Can you work these out from the model? Positions are in its coordinate system, mm. Face numbers are marked on the shaded views. A direction names the side the tool comes from. Coordinates: 2 decimals unless noted, no trailing zeros. Loops run counter-clockwise (first coordinate to the right, second up) from the corner with the lowest first, then second, coordinate; pieces in that order, holes last. Notation, with made-up numbers: (5.5, -0.5) -> (24.5, -0.5) arc R14 ccw to (24.5, 6.5) -> close; hole circle Ø1 at (29, -14). An arc over 180 degrees is marked (long way). Use one line per item in the form item = value. Start each with the question number.
(1) Imagine slicing it at B-B (y = 18). List the corners of the cut face in (x, z) for me, plus the area to 3 significant figures.
(2) Imagine slicing it at D-D (z = 17.5). List the corners of the cut face in (x, y) for me.
(3) Imagine slicing it at C-C (x = 33). List the corners of the cut face in (y, z) for me.
(4) On a 3-axis mill with a long thin cutter (end or side, diameter ignored), from which of +Z, -Z, +X, -X, +Y, -Y can I reach the whole of each face in a straight line? I mean the marked faces 1 and 2. Say none if no direction works.
(5) I need wall thicknesses on line 1 (X direction, y = 0.65, z = 33); line 2 (Z direction, x = 8, y = 1); line 3 (Y direction, x = 24.5, z = 29.5). Which ranges of each line are inside material? Lowest first, please. Write a range as [from, to].
(6) I'm going to push flat-ended pins straight in: pin 1 (10 mm diameter, centred on y = 14, z = 35.5, fed in from +X); pin 2 (5 mm diameter, centred on x = 33, z = 7, fed in from +Y); pin 3 (2.5 mm diameter, centred on x = 33, z = 33, fed in from -Y). Where does each tip first touch, or does it pass through?
(7) Imagine slicing it at A-A (z = 33). List the corners of the cut face in (x, y) for me.
```python
from build123d import *

# Parameters (mm, degrees)
EXTRUSION1_DEPTH = 40
ESQUISSE2_R      = 6.5
EXTRUSION2_DEPTH = 30
ESQUISSE3_R      = 1.5
EXTRUSION3_DEPTH = 30


with BuildPart() as part:
    # Esquisse1 → Extrusion1 (new body)
    with BuildSketch(Plane.XY):
        Polygon((0, 0), (0, 40), (1.5, 40), (1.5, 1.5), (40, 1.5), (40, 0), align=None)
    extrude(amount=EXTRUSION1_DEPTH)

    # Esquisse2 → Extrusion2 (cut)
    with BuildSketch(Plane(origin=(1.5, 0, 0), x_dir=(0, 0, -1), z_dir=(1, 0, 0))):
        with Locations(Location((-20, 18, 0), (0, 0, 90))):
            Circle(ESQUISSE2_R)
    extrude(amount=-EXTRUSION2_DEPTH, mode=Mode.SUBTRACT)

    # Esquisse3 → Extrusion3 (cut)
    with BuildSketch(Plane(origin=(0, 1.5, 0), x_dir=(-1, 0, 0), z_dir=(0, 1, 0))):
        with Locations(Location((-8.5, 33, 0), (0, 0, 90))):
            Circle(ESQUISSE3_R)
        with Locations(Location((-8.5, 7, 0), (0, 0, 90))):
            Circle(ESQUISSE3_R)
        with Locations(Location((-33, 7, 0), (0, 0, 90))):
            Circle(ESQUISSE3_R)
        with Locations(Location((-33, 33, 0), (0, 0, 90))):
            Circle(ESQUISSE3_R)
    extrude(amount=-EXTRUSION3_DEPTH, mode=Mode.SUBTRACT)


solid = part.part
```
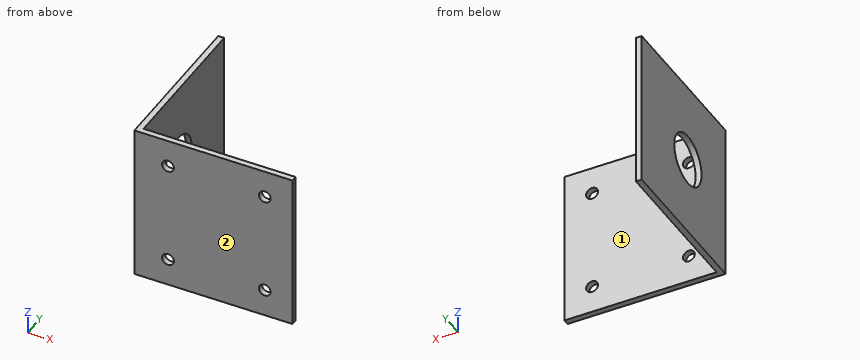
Worked out:
q1.outline = (0, 0) -> (1.5, 0) -> (1.5, 13.5) -> (0, 13.5) -> close; (0, 26.5) -> (1.5, 26.5) -> (1.5, 40) -> (0, 40) -> close
q1.area = 40.5 mm2
q2.outline = (0, 0) -> (40, 0) -> (40, 1.5) -> (1.5, 1.5) -> (1.5, 12) -> (0, 12) -> close; (0, 24) -> (1.5, 24) -> (1.5, 40) -> (0, 40) -> close
q3.outline = (0, 0) -> (1.5, 0) -> (1.5, 5.5) -> (0, 5.5) -> close; (0, 8.5) -> (1.5, 8.5) -> (1.5, 31.5) -> (0, 31.5) -> close; (0, 34.5) -> (1.5, 34.5) -> (1.5, 40) -> (0, 40) -> close
q4.face_1 = +Z, -Z, +X, +Y
q4.face_2 = +Z, -Z, +X, -X, -Y
q5.line_1 = [0, 7], [10, 31.5], [34.5, 40]
q5.line_2 = [0, 5.59], [8.41, 31.59], [34.41, 40]
q5.line_3 = [0, 1.5]
q6.pin_1 = 1.5
q6.pin_2 = 1.5
q6.pin_3 = through
q7.outline = (0, 0) -> (7, 0) -> (7, 1.5) -> (1.5, 1.5) -> (1.5, 40) -> (0, 40) -> close; (10, 0) -> (31.5, 0) -> (31.5, 1.5) -> (10, 1.5) -> close; (34.5, 0) -> (40, 0) -> (40, 1.5) -> (34.5, 1.5) -> close
